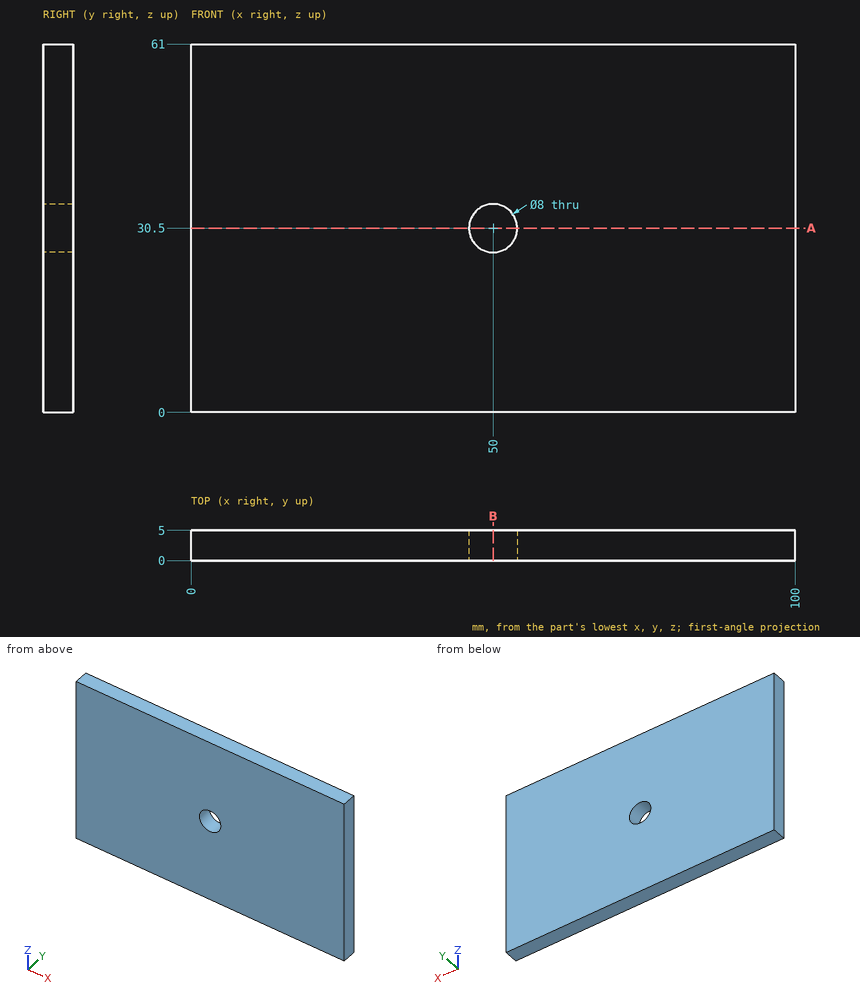
Job drawing, mm, ordinate dimensions from the low corner. One solid piece. Coordinates: 2 decimals unless noted, no trailing zeros. Loops run counter-clockwise (first coordinate to the right, second up) from the corner with the lowest first, then second, coordinate; pieces in that order, holes last. Notation, with made-up numbers: (-19.75, 38.5) -> (-2.75, 38.5) arc R28 ccw to (-2.75, 66.5) -> close; hole circle Ø8 at (13, 7). An arc over 180 degrees is marked (long way). One line per item, written item: value.
1. Drill centre lines: line 1 (X direction, y = 3.95, z = 30.5); line 2 (Z direction, x = 50, y = 2.4); line 3 (X direction, y = 3.15, z = 32). Where is each one in solid material? Low to high. Write a range as [from, to].
Answers:
line 1: x = [0, 46], [54, 100]
line 2: z = [0, 26.5], [34.5, 61]
line 3: x = [0, 46.29], [53.71, 100]
2. Flat gauge pin, fed straight in: P1, Ø6, axis at x = 24, z = 51.5, coming from the -Y side. Where does the tip first touch, or does it go through?
Answers:
P1: stops at y = 0
3. Slice it at A-A on z = 30.5. Write the cut outline in (x, y), and give its area (3 significant figures).
Answers:
outline: (0, 0) -> (46, 0) -> (46, 5) -> (0, 5) -> close; (54, 0) -> (100, 0) -> (100, 5) -> (54, 5) -> close
area: 460 mm^2
4. Slice it at B-B on x = 50. Write the cut outline in (y, z).
Answers:
outline: (0, 0) -> (5, 0) -> (5, 26.5) -> (0, 26.5) -> close; (0, 34.5) -> (5, 34.5) -> (5, 61) -> (0, 61) -> close
